```python
from build123d import *

# Parameters (mm, degrees)
SKETCH1_R                = 8.5
BOSS_EXTRUDE1_DEPTH      = 70
BOSS_EXTRUDE1_DEPTH_BACK = 70
SKETCH2_R                = 10
BOSS_EXTRUDE2_DEPTH      = 37
BOSS_EXTRUDE2_DEPTH_BACK = 37


with BuildPart() as part:
    # Sketch1 → Boss-Extrude1 (new body, two sides)
    with BuildSketch(Plane(origin=(0, 0, 0), x_dir=(1, 0, 0), z_dir=(0, 1, 0))) as boss_extrude1_sk:
        Circle(SKETCH1_R)
    extrude(amount=BOSS_EXTRUDE1_DEPTH)
    extrude(boss_extrude1_sk.sketch, amount=-BOSS_EXTRUDE1_DEPTH_BACK)

    # Sketch2 → Boss-Extrude2 (add, two sides)
    with BuildSketch(Plane(origin=(0, 0, 0), x_dir=(1, 0, 0), z_dir=(0, 1, 0))) as boss_extrude2_sk:
        Circle(SKETCH2_R)
    extrude(amount=BOSS_EXTRUDE2_DEPTH)
    extrude(boss_extrude2_sk.sketch, amount=-BOSS_EXTRUDE2_DEPTH_BACK)


solid = part.part
```
Geometry: final body of the model. Coordinates: model frame, mm. A direction names the side the tool comes from. Round coordinates to 2 decimals unless told otherwise and drop trailing zeros. Order: outer loops, then holes, each group sorted by start corner. A loop starts at its lowest first (then second) coordinate and runs counter-clockwise, first axis right, second up. Notation, with made-up numbers: (-30, 24) -> (3, 24) arc R20 cw to (3, 43) -> close; hole circle Ø6 at (-24.75, 47.25). An arc over 180 degrees is marked (long way). Use one line per item in the form item = value. Start each with the question number.
1. Line query: probe 1 along Z at (x, y) = (-5.25, -3.5); probe 2 along Y at (x, z) = (7.25, 5.5); probe 3 along X at (y, z) = (53.5, -0.25). Output: solid intervals per line, ascending.
2. Pin query (flat end, axial travel): pin 1 Ø1 at (x, y) = (-2, -27) entering from +Z; pin 2 Ø1.5 at (y, z) = (49, -2) entering from -X; pin 3 Ø10 at (y, z) = (53.5, -2) entering from -X. Return the tip coordinate at first contact, or that it passes through.
3. Cut plane D-D (y = 1.5). Return the cut outline in (x, z), then the cut area to 3 significant figures.
4. Cut plane C-C (y = -48). Return the cut outline in (x, z), then the cut area to 3 significant figures.
5. Cut plane B-B (x = 1.25). Return the cut outline in (y, z), then the cut area to 3 significant figures.
6. Reachability of faces 1 (the face through (4.57, -53.269, -7.167)), 2 (the face through (-4.5, 37, 7.4)), 3 (the face through (0, 70, 0)) from +Z, -Z, +X, -X, +Y, -Y: full face, straight path, thin tool, end or side. Return the list, or none.
7. Cut plane A-A (z = 0). Return the cut outline in (x, y), then the cut area to 3 significant figures.
Solution:
q1.probe_1 = -8.51 to 8.51
q1.probe_2 = -37 to 37
q1.probe_3 = -8.5 to 8.5
q2.pin_1 = 9.89
q2.pin_2 = -8.41
q2.pin_3 = -8.5
q3.outline = circle Ø20 at (0, 0)
q3.area = 314 mm^2
q4.outline = circle Ø17 at (0, 0)
q4.area = 227 mm^2
q5.outline = (-70, -8.41) -> (-37, -8.41) -> (-37, -9.92) -> (37, -9.92) -> (37, -8.41) -> (70, -8.41) -> (70, 8.41) -> (37, 8.41) -> (37, 9.92) -> (-37, 9.92) -> (-37, 8.41) -> (-70, 8.41) -> close
q5.area = 2,580 mm^2
q6.face_1 = -Y
q6.face_2 = +Y
q6.face_3 = +Z, -Z, +X, -X, +Y
q7.outline = (-10, -37) -> (-8.5, -37) -> (-8.5, -70) -> (8.5, -70) -> (8.5, -37) -> (10, -37) -> (10, 37) -> (8.5, 37) -> (8.5, 70) -> (-8.5, 70) -> (-8.5, 37) -> (-10, 37) -> close
q7.area = 2,600 mm^2
